Source: CAD feature listing. Evaluate the final solid. Frame: model axes, mm. Face numbers are marked on the shaded views. A direction names the side the tool comes from. Give positions to 0.01 mm unless a question says otherwise; leave off trailing zeros. Order: outer loops, then holes, each group sorted by start corner. A loop starts at its lowest first (then second) coordinate and runs counter-clockwise, first axis right, second up.
from build123d import *

# Parameters (mm, degrees)
SKETCH1_W           = 20
SKETCH1_H           = 20
BOSS_EXTRUDE1_DEPTH = 10
SKETCH2_W           = 10
SKETCH2_H           = 10
BOSS_EXTRUDE2_DEPTH = 30
SKETCH3_W           = 5
SKETCH3_H           = 2
BOSS_EXTRUDE3_DEPTH = 3
SKETCH4_R           = 2.5
BOSS_EXTRUDE4_DEPTH = 2


with BuildPart() as part:
    # Sketch1 → Boss-Extrude1 (new body)
    with BuildSketch(Plane(origin=(0, 0, 0), x_dir=(1, 0, 0), z_dir=(0, 1, 0))):
        Rectangle(SKETCH1_W, SKETCH1_H)
    extrude(amount=BOSS_EXTRUDE1_DEPTH)

    # Sketch2 → Boss-Extrude2 (add)
    with BuildSketch(Plane(origin=(0, 0, 0), x_dir=(-1, 0, 0), z_dir=(0, -1, 0))):
        Rectangle(SKETCH2_W, SKETCH2_H)
    extrude(amount=BOSS_EXTRUDE2_DEPTH)

    # Sketch3 → Boss-Extrude3 (add)
    with BuildSketch(Plane(origin=(0, -30, 0), x_dir=(-1, 0, 0), z_dir=(0, -1, 0))):
        with Locations((0, 4)):
            Rectangle(SKETCH3_W, SKETCH3_H)
        with Locations((0, -4)):
            Rectangle(SKETCH3_W, SKETCH3_H)
    extrude(amount=BOSS_EXTRUDE3_DEPTH)

    # Sketch4 → Boss-Extrude4 (add)
    with BuildSketch(Plane(origin=(0, 0, -5), x_dir=(1, 0, 0), z_dir=(0, 0, -1))):
        with Locations((0, 33)):
            Circle(SKETCH4_R)
    boss_extrude4 = extrude(amount=-BOSS_EXTRUDE4_DEPTH)

    # Mirror2: Boss-Extrude4 across plane
    add(boss_extrude4.mirror(Plane.XY))


solid = part.part
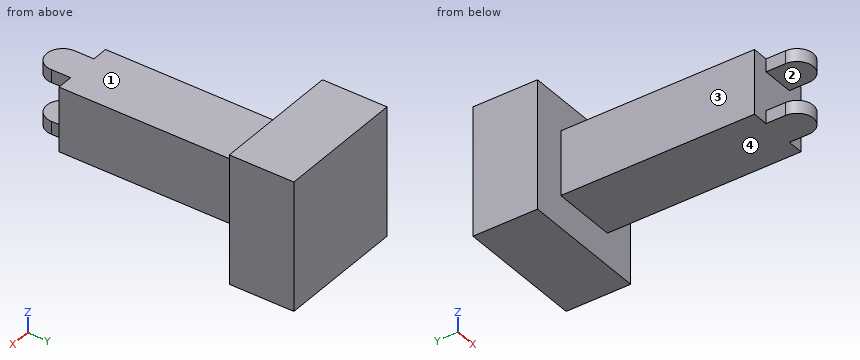
1) Section query D-D on y = -3. Output: boundary loops of the cut face in (x, z), and give its area (3 significant figures).
Checks:
outline: (-5, -5) - (5, -5) - (5, 5) - (-5, 5) - close
area: 100 mm2
2) First-contact query: pin 1 Ø1.6 at (y, z) = (-32, 4.5) entering from -X; pin 2 Ø4 at (y, z) = (-18.5, 3.5) entering from +X; pin 3 Ø1.5 at (x, z) = (-3, 7) entering from -Y. Flat tips, straight axial feed; report the tip coordinate or a pass-through.
Checks:
pin 1: stops at x = -2.5
pin 2: stops at x = 5
pin 3: stops at y = 0
3) Section query C-C on z = 2. Output: boundary loops of the cut face in (x, y).
Checks:
outline: (-10, 0) - (-5, 0) - (-5, -30) - (5, -30) - (5, 0) - (10, 0) - (10, 10) - (-10, 10) - close
4) Section query A-A on z = -4. Output: boundary loops of the cut face in (x, y), and give its area (3 significant figures).
Checks:
outline: (-10, 0) - (-5, 0) - (-5, -30) - (-2.5, -30) - (-2.5, -33) arc R2.5 ccw to (2.5, -33) - (2.5, -30) - (5, -30) - (5, 0) - (10, 0) - (10, 10) - (-10, 10) - close
area: 525 mm2
5) Ray query, L1, parallel to Z at x = -2, y = -10; L2, parallel to Y at x = 6.5, z = 4.75. Return the intervals inside material, ascending.
Checks:
L1: z = -5 to 5
L2: y = 0 to 10
6) Reachability of the marked faces 1, 2, 3 and 4 from +Z, -Z, +X, -X, +Y, -Y: full face, straight path, thin tool, end or side. Return the list, or none.
Checks:
face 1: +Z, +X, -X, -Y
face 2: +X, -X, -Y
face 3: +Z, -Z, -X, -Y
face 4: -Z, +X, -X, -Y
7) Section query B-B on x = 1.5. Output: boundary loops of the cut face in (y, z).
Checks:
outline: (-35, -5) - (0, -5) - (0, -10) - (10, -10) - (10, 10) - (0, 10) - (0, 5) - (-35, 5) - (-35, 3) - (-30, 3) - (-30, -3) - (-35, -3) - close
